Read the model definition and answer for the solid it produces. Units are mm, in the model's axes. A direction names the side the tool comes from. Round coordinates to 2 decimals unless told otherwise and drop trailing zeros. Write each loop counter-clockwise with the first axis right and the second up, starting at its lowest first coordinate (ties: lowest second). Pieces come first, ordered by that corner, then holes.
from build123d import *

# Parameters (mm, degrees)
SKETCH1_R           = 40
BOSS_EXTRUDE1_DEPTH = 30
SKETCH2_W           = 80
SKETCH2_H           = 80
SKETCH2_R           = 2.5
BOSS_EXTRUDE2_DEPTH = 3
FILLET1_R           = 4
SKETCH3_R           = 34
BOSS_EXTRUDE3_DEPTH = 100
FILLET2_R           = 4
SKETCH4_R           = 5
BOSS_EXTRUDE4_DEPTH = 50
FILLET3_R           = 1
SKETCH5_W           = 42.68943546
SKETCH5_H           = 2
CUT_EXTRUDE1_DEPTH  = 81


with BuildPart() as part:
    # Sketch1 → Boss-Extrude1 (new body)
    with BuildSketch(Plane.XY):
        Circle(SKETCH1_R)
    extrude(amount=BOSS_EXTRUDE1_DEPTH)

    # Sketch2 → Boss-Extrude2 (add)
    with BuildSketch(Plane.XY.offset(30)):
        Rectangle(SKETCH2_W, SKETCH2_H)
        with Locations((33, -33)):
            Circle(SKETCH2_R, mode=Mode.SUBTRACT)
        with Locations((-33, 33)):
            Circle(SKETCH2_R, mode=Mode.SUBTRACT)
        with Locations((33, 33)):
            Circle(SKETCH2_R, mode=Mode.SUBTRACT)
        with Locations((-33, -33)):
            Circle(SKETCH2_R, mode=Mode.SUBTRACT)
    extrude(amount=BOSS_EXTRUDE2_DEPTH)

    # Fillet1
    fillet1_edges = [part.edges().sort_by_distance(p)[0] for p in [
        (40, 40, 31.5),
        (-40, 40, 31.5),
        (-40, -40, 31.5),
        (40, -40, 31.5),
    ]]
    fillet(fillet1_edges, radius=FILLET1_R)

    # Sketch3 → Boss-Extrude3 (add)
    with BuildSketch(Plane(origin=(0, 0, 0), x_dir=(-1, 0, 0), z_dir=(0, 0, -1))):
        Circle(SKETCH3_R)
    extrude(amount=BOSS_EXTRUDE3_DEPTH)

    # Fillet2
    fillet2_edges = [part.edges().sort_by_distance(p)[0] for p in [
        (-40, 0, 0),
        (34, 0, -100),
    ]]
    fillet(fillet2_edges, radius=FILLET2_R)

    # Sketch4 → Boss-Extrude4 (add)
    with BuildSketch(Plane.XY.offset(33)):
        with Locations((0, -14)):
            Circle(SKETCH4_R)
    extrude(amount=BOSS_EXTRUDE4_DEPTH)

    # Fillet3
    fillet3_edges = [part.edges().sort_by_distance(p)[0] for p in [
        (-5, -14, 83),
    ]]
    fillet(fillet3_edges, radius=FILLET3_R)

    # Sketch5 → Cut-Extrude1 (cut, through all)
    with BuildSketch(Plane.ZY.offset(40)):
        with Locations((64.34471773, -10)):
            Rectangle(SKETCH5_W, SKETCH5_H)
    extrude(amount=-CUT_EXTRUDE1_DEPTH, mode=Mode.SUBTRACT)


solid = part.part
Q1. Determine the mould class of faces 5 (the flat face through (-30, -30, 30)), 6 (the cylindrical face through (32.67, -30.52, 31.48)), 7 (the cylindrical face through (34.34, 35.11, 31.48)), 8 (the cylindrical face through (2.307, -18.436, 57.157)) for opening direction X: pulls with the +X half, pulls with the -X half, needs draft (parallel to the pull), parting line crosses it, or undercut.
Verdict:
face 5: needs draft
face 6: undercut
face 7: undercut
face 8: parting line crosses it
Q2. Straight lines are drawn through the part: probe 1 along Y at (x, z) = (33, 31.25); probe 2 along Z at (x, y) = (-18, -21.5); probe 3 along Y at (x, z) = (0.5, -40.5). For each, find the intervals that lie inside material, in ascending order.
Verdict:
probe 1: y = -40 to -35.5, -30.5 to 30.5, 35.5 to 40
probe 2: z = -100 to 33
probe 3: y = -34 to 34
Q3. Section A-A (z = -21.5) is taken. Determine the outline of the cut face in (x, y), then the cut area to 3 significant figures.
Verdict:
outline: circle Ø68 at (0, 0)
area: 3,630 mm2
Q4. Section C-C (z = 47) is taken. Determine the outline of the cut face in (x, y), then the cut area to 3 significant figures.
Verdict:
outline: (-4, -11) arc R5 ccw (long way) to (4, -11) - close
area: 67.4 mm2
Q5. Section B-B (z = 13) is taken. Determine the outline of the cut face in (x, y), then the cut area to 3 significant figures.
Verdict:
outline: circle Ø80 at (0, 0)
area: 5,030 mm2
Q6. Flat-ended cylindrical pins translate along their axes: pin 1 Ø1 at (y, z) = (-25, -63) entering from -X; pin 2 Ø2 at (x, z) = (-6.5, 21) entering from +Y; pin 3 Ø6 at (x, z) = (28, -60.5) entering from -Y. Find the tip coordinate at first contact, or state that the pin passes through.
Verdict:
pin 1: stops at x = -23.57
pin 2: stops at y = 39.62
pin 3: stops at y = -23.04
Q7. Which of the six approach directions +Z, -Z, +X, -X, +Y, -Y give full straight-line access (tool end or side, diameter ignored) to faces 1 (the flat face through (30, 32, 30)), 2 (the flat face through (-30, 32, 30)), 3 (the flat face through (0, -11, 63)), 4 (the flat face through (32, -13, 0))?
Verdict:
face 1: -Z, +X, +Y
face 2: -Z, -X, +Y
face 3: +Z, +X, -X, +Y
face 4: -Z
